Verification items for the finished model (mm, model axes). Coordinates: 2 decimals unless noted, no trailing zeros. Write each loop counter-clockwise with the first axis right and the second up, starting at its lowest first coordinate (ties: lowest second). Pieces come first, ordered by that corner, then holes. Notation, with made-up numbers: (-5, 68) -> (29, 68) arc R23 cw to (29, 90) -> close; hole circle Ø6 at (44.5, 15.5). An arc over 180 degrees is marked (long way). Answer in a Markdown table with one row per item.
```python
from build123d import *

# Parameters (mm, degrees)
F0_W     = 540
F0_H     = 440
F0_W_2   = 504
F0_H_2   = 404
F0_W_3   = 490
F0_H_3   = 390
F1_DEPTH = 3
F2_DEPTH = 10


with BuildPart() as f1:
    # F0 (on Top) → F1 (new body)
    with BuildSketch(Plane.XY):
        Rectangle(F0_W, F0_H)
        Rectangle(F0_W_2, F0_H_2, mode=Mode.SUBTRACT)
        Rectangle(F0_W_2, F0_H_2)
        Rectangle(F0_W_3, F0_H_3, mode=Mode.SUBTRACT)
    extrude(amount=-F1_DEPTH)

    # F0 (on Top) → F2 (join)
    with BuildSketch(Plane.XY):
        Rectangle(F0_W, F0_H)
        Rectangle(F0_W_2, F0_H_2, mode=Mode.SUBTRACT)
    extrude(amount=-F2_DEPTH)


solid = f1.part
```
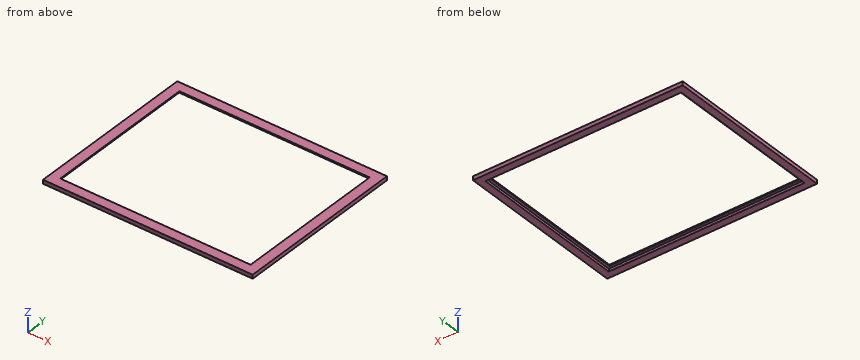
1. Thickness scan on line 1 (Y direction, x = 210, z = -6.75); line 2 (X direction, y = 152, z = -4); line 3 (Y direction, x = 80.5, z = -2.25). Record the ranges inside material, lowest first. Write a range as from..to.
Geometry says:
| item | result |
|---|---|
| line 1 | -220..-202, 202..220 |
| line 2 | -270..-252, 252..270 |
| line 3 | -220..-195, 195..220 |
2. Section check B-B, the plane y = 49. Record the boundary of the cut face in (x, z).
Geometry says:
| item | result |
|---|---|
| outline | (-270, -10) -> (-252, -10) -> (-252, -3) -> (-245, -3) -> (-245, 0) -> (-270, 0) -> close; (245, -3) -> (252, -3) -> (252, -10) -> (270, -10) -> (270, 0) -> (245, 0) -> close |
3. Section check C-C, the plane z = -7.75. Record the boundary of the cut face in (x, y).
Geometry says:
| item | result |
|---|---|
| outline | (-270, -220) -> (270, -220) -> (270, 220) -> (-270, 220) -> close; hole (-252, -202) -> (252, -202) -> (252, 202) -> (-252, 202) -> close |
4. Section check A-A, the plane x = -115. Record the boundary of the cut face in (y, z), plus the area to 3 significant figures.
Geometry says:
| item | result |
|---|---|
| outline | (-220, -10) -> (-202, -10) -> (-202, -3) -> (-195, -3) -> (-195, 0) -> (-220, 0) -> close; (195, -3) -> (202, -3) -> (202, -10) -> (220, -10) -> (220, 0) -> (195, 0) -> close |
| area | 402 mm^2 |
